Geometry: see drawing. Coordinates: mm, zero at the bounding-box minimum. A direction names the side the tool comes from. Give positions to 0.01 mm unless a question says otherwise; leave off trailing zeros. Write each loop counter-clockwise with the first axis right and the second up, starting at its lowest first coordinate (ties: lowest second). Pieces come first, ordered by that corner, then holes. Notation, with made-up numbers: (24, 20) -> (69, 20) arc R19 ccw to (69, 57) -> close; hole circle Ø10 at (-24.75, 69.25). An arc over 180 degrees is marked (long way). Write item = value, one per line.
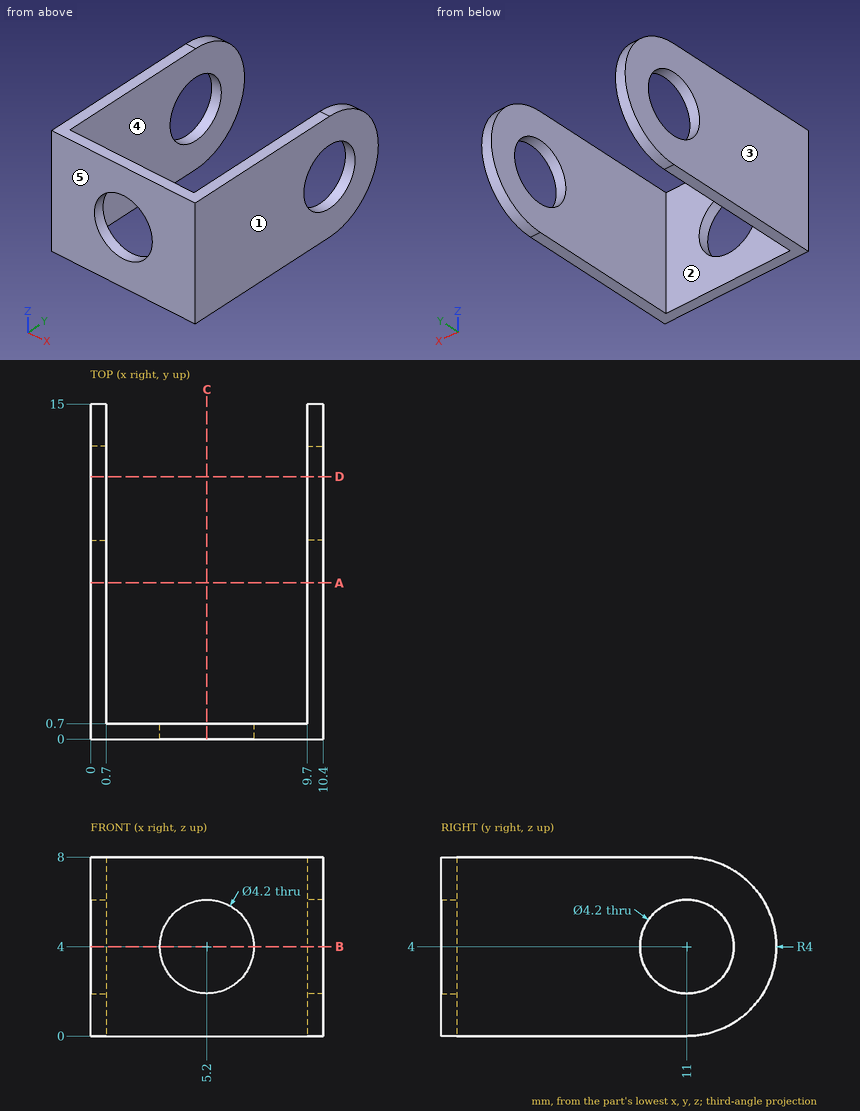
(1) Pull-direction query (X, two-part tool) for the marked faces 1, 2 and 3; classes: pulls with the +X half, pulls with the -X half, needs draft (parallel to the pull), parting line crosses it, or undercut.
Values follow:
face_1 = pulls with the +X half
face_2 = undercut
face_3 = pulls with the -X half
(2) Section query C-C (x = 5.2). Return loops of the section in (y, z), plus the area to 3 significant figures.
Values follow:
outline = (0, 0) -> (0.7, 0) -> (0.7, 1.9) -> (0, 1.9) -> close; (0, 6.1) -> (0.7, 6.1) -> (0.7, 8) -> (0, 8) -> close
area = 2.66 mm2
(3) First-contact query: pin 1 (1 mm diameter, centred on x = 7.5, z = 6, fed in from +Y); pin 2 (4 mm diameter, centred on x = 3.5, y = 11, fed in from +Z). Flat tips, straight axial feed; report the tip coordinate or a pass-through.
Values follow:
pin_1 = 0.7
pin_2 = through
(4) Section query B-B (z = 4). Return loops of the section in (x, y).
Values follow:
outline = (0, 0) -> (3.1, 0) -> (3.1, 0.7) -> (0.7, 0.7) -> (0.7, 8.9) -> (0, 8.9) -> close; (0, 13.1) -> (0.7, 13.1) -> (0.7, 15) -> (0, 15) -> close; (7.3, 0) -> (10.4, 0) -> (10.4, 8.9) -> (9.7, 8.9) -> (9.7, 0.7) -> (7.3, 0.7) -> close; (9.7, 13.1) -> (10.4, 13.1) -> (10.4, 15) -> (9.7, 15) -> close
(5) Material intervals for line 1 (X direction, y = 0.4, z = 4); line 2 (X direction, y = 9.5, z = 7.75); line 3 (Z direction, x = 10.25, y = 11), sorted ascending.
Values follow:
line_1 = 0 to 3.1, 7.3 to 10.4
line_2 = 0 to 0.7, 9.7 to 10.4
line_3 = 0 to 1.9, 6.1 to 8
(6) Section query A-A (y = 7). Return loops of the section in (x, z), plus the area to 3 significant figures.
Values follow:
outline = (0, 0) -> (0.7, 0) -> (0.7, 8) -> (0, 8) -> close; (9.7, 0) -> (10.4, 0) -> (10.4, 8) -> (9.7, 8) -> close
area = 11.2 mm2
(7) Section query D-D (y = 11.75). Return loops of the section in (x, z), plus the area to 3 significant figures.
Values follow:
outline = (0, 0.07) -> (0.7, 0.07) -> (0.7, 2.04) -> (0, 2.04) -> close; (0, 5.96) -> (0.7, 5.96) -> (0.7, 7.93) -> (0, 7.93) -> close; (9.7, 0.07) -> (10.4, 0.07) -> (10.4, 2.04) -> (9.7, 2.04) -> close; (9.7, 5.96) -> (10.4, 5.96) -> (10.4, 7.93) -> (9.7, 7.93) -> close
area = 5.51 mm2
(8) Access query for the marked faces 4 and 5. Directions: +Z, -Z, +X, -X, +Y, -Y. A direction counts if a zero-diameter tool reaches every point of the face in a straight line with its end or side. Return the directions, or none.
Values follow:
face_4 = +Z, -Z, +Y
face_5 = +Z, -Z, +X, -X, -Y
